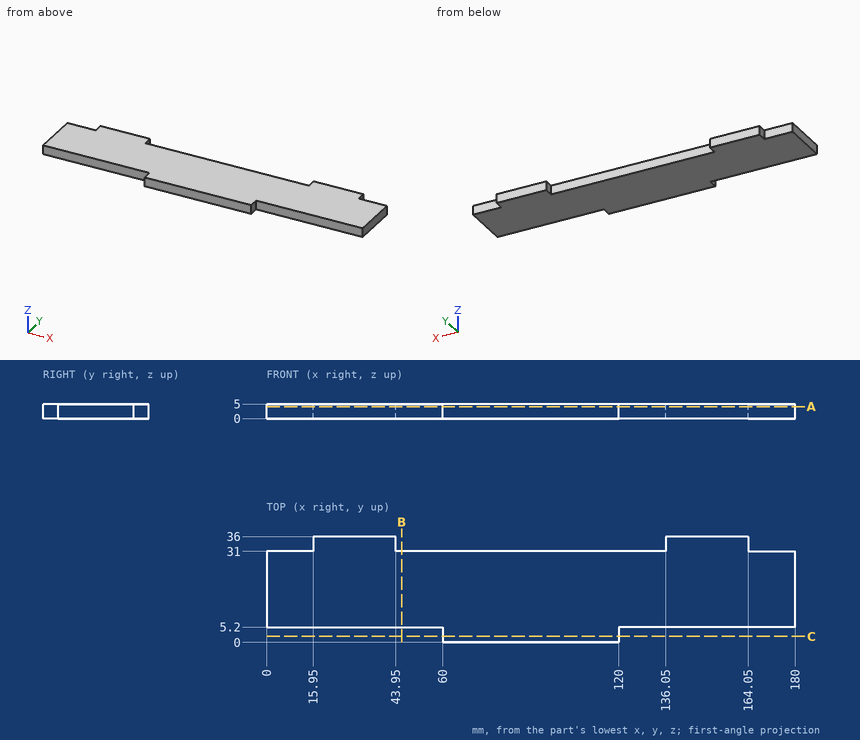
The figure shows three views and two pictorial views of one solid part (mm, origin at its lowest corner). Answer the questions. Give positions to 0.01 mm unless a question says otherwise; leave off trailing zeros. Order: outer loops, then holes, each group sorted by start corner. A loop starts at its lowest first (then second) coordinate and runs counter-clockwise, first axis right, second up. Notation, with made-up numbers: (51, 74) -> (86, 74) arc R17 cw to (86, 79) -> close; hole circle Ø9 at (17.25, 86.5). An arc over 180 degrees is marked (long way). One line per item, written item: value.
1) Find section A-A, the plane z = 4.1. Determine the outline of the cut face in (x, y).
Reported:
outline: (0, 5.2) -> (60, 5.2) -> (60, 0) -> (120, 0) -> (120, 5.2) -> (180, 5.2) -> (180, 31) -> (164.05, 31) -> (164.05, 36) -> (136.05, 36) -> (136.05, 31) -> (43.95, 31) -> (43.95, 36) -> (15.95, 36) -> (15.95, 31) -> (0, 31) -> close
2) Find section B-B, the plane x = 46. Determine the outline of the cut face in (y, z).
Reported:
outline: (5.2, 0) -> (31, 0) -> (31, 5) -> (5.2, 5) -> close
3) Find the intervals of material crossed by line 1 (Y direction, x = 111, z = 2); line 2 (Y direction, x = 8, z = 2.1); line 3 (X direction, y = 2.5, z = 1.9), in increasing order.
Reported:
line 1: y = 0 to 31
line 2: y = 5.2 to 31
line 3: x = 60 to 120
4) Flat-ended cylindrical pins translate along their axes: P1, Ø2.5, axis at y = 32.5, z = 3.5, coming from the +X side; P2, Ø1.5, axis at x = 5.5, z = 3.5, coming from the +Y side; P3, Ø1.5, axis at x = 159.5, z = 2, coming from the -Y side. Find the tip coordinate at first contact, or state that the pin passes through.
Reported:
P1: stops at x = 164.05
P2: stops at y = 31
P3: stops at y = 5.2
5) Find section C-C, the plane y = 2. Determine the outline of the cut face in (x, z), plus the area to 3 significant figures.
Reported:
outline: (60, 0) -> (120, 0) -> (120, 5) -> (60, 5) -> close
area: 300 mm^2
